Geometry: final body of the model. Coordinates: model frame, mm. A direction names the side the tool comes from. Round coordinates to 2 decimals unless told otherwise and drop trailing zeros. Loops run counter-clockwise (first coordinate to the right, second up) from the corner with the lowest first, then second, coordinate; pieces in that order, holes last. Notation, with made-up numbers: (49.5, 5) - (73.5, 5) arc R20 ccw to (73.5, 40) - close; hole circle Ø2 at (87.5, 49.25). An arc over 180 degrees is marked (long way). Answer as a JSON object with one key per item and string values. Group by question number.
Item 1: Section B-B (y = 0). Return the cut outline in (x, z) (3 decimals), plus the area to 3 significant figures.
Item 2: Section A-A (z = -10.5). Return the cut outline in (x, y).
Item 3: First-contact query: pin 1 (4.5 mm diameter, centred on y = 0, z = 0, fed in from -X); pin 2 (3 mm diameter, centred on x = 15, y = -0.5, fed in from +Z). Flat tips, straight axial feed; report the tip coordinate or a pass-through.
Item 4: Section C-C (y = -6.5). Return the cut outline in (x, z), plus the area to 3 significant figures.
Item 5: Draft query along Y for faces 4 (the face through (19, -9.596, -6)), 5 (the face through (19, -12.596, 8)), 6 (the face through (19, 12.596, -8)). Return one class per face: released by +Y, released by -Y, zero draft, split by the parting line, or undercut.
Item 6: Line query: line 1 (Z direction, x = 9.5, y = -10.25); line 2 (Z direction, x = 34, y = -7); line 3 (Y direction, x = 18, z = 0) (3 decimals). Output: solid intervals per line, ascending.
Item 7: Reachability of faces 1 (the face through (18.783, 7.495, -5.049)), 2 (the face through (19, 5, 0)), 3 (the face through (19, -11, 3.24)) from +Z, -Z, +X, -X, +Y, -Y: full face, straight path, thin tool, end or side. Return the list, or none.
```python
from build123d import *

# Parameters (mm, degrees)
SKETCH1_W           = 10
SKETCH1_H           = 10
SKETCH1_R           = 2.605
BOSS_EXTRUDE1_DEPTH = 38.1
CIRPATTERN1_COUNT   = 4


with BuildPart() as part:
    # Sketch1 → Boss-Extrude1 (new body)
    with BuildSketch(Plane(origin=(0, 0, 0), x_dir=(0, 0, -1), z_dir=(1, 0, 0))):
        Rectangle(SKETCH1_W, SKETCH1_H)
        Circle(SKETCH1_R, mode=Mode.SUBTRACT)
        Polygon((7.474873734, 9.921463197), (2.553410537, 5), (5, 5), (5, 3.203948776), (9.596194078, 7.800142853), align=None)
        Polygon((9.596194078, 3.24), (12.596194078, 3.24), (12.596194078, 12.596194078), (3.24, 12.596194078), (3.24, 9.921463197), (7.474873734, 9.921463197), (9.596194078, 7.800142853), align=None)
    boss_extrude1 = extrude(amount=BOSS_EXTRUDE1_DEPTH)

    # CirPattern1: Boss-Extrude1 ×4 about axis
    cirpattern1_axis = Axis((0, 0, 0), (1, 0, 0))
    for i in range(1, CIRPATTERN1_COUNT):
        add(boss_extrude1.rotate(cirpattern1_axis, i * 360 / CIRPATTERN1_COUNT))


solid = part.part
```
Values:
{
 "1": {"outline": "(0, -5) - (38.1, -5) - (38.1, -2.605) - (0, -2.605) - close; (0, 2.605) - (38.1, 2.605) - (38.1, 5) - (0, 5) - close", "area": "182 mm^2"},
 "2": {"outline": "(0, -12.6) - (38.1, -12.6) - (38.1, -3.24) - (0, -3.24) - close; (0, 3.24) - (38.1, 3.24) - (38.1, 12.6) - (0, 12.6) - close"},
 "3": {"pin 1": "passes through", "pin 2": "stops at z = 5"},
 "4": {"outline": "(0, -12.6) - (38.1, -12.6) - (38.1, -9.92) - (0, -9.92) - close; (0, -8.95) - (38.1, -8.95) - (38.1, -4.7) - (0, -4.7) - close; (0, 4.05) - (38.1, 4.05) - (38.1, 8.3) - (0, 8.3) - close; (0, 9.6) - (38.1, 9.6) - (38.1, 12.6) - (0, 12.6) - close", "area": "539 mm^2"},
 "5": {"face 4": "undercut", "face 5": "released by -Y", "face 6": "released by +Y"},
 "6": {"line 1": "z = -12.6 to -3.24, 3.24 to 12.6", "line 2": "z = -12.6 to -9.92, -9.45 to -5.2, 4.55 to 8.8, 9.6 to 12.6", "line 3": "y = -5 to -2.605, 2.605 to 5"},
 "7": {"face 1": "+X, -X", "face 2": "+X, -X, +Y", "face 3": "+X, -X, -Y"}
}
